Check sheet for the modelled part. Datum: model origin and axes. Units: mm. A direction names the side the tool comes from. Give positions to 0.01 mm unless a question says otherwise; leave off trailing zeros. Order: outer loops, then holes, each group sorted by start corner. A loop starts at its lowest first (then second) coordinate and runs counter-clockwise, first axis right, second up. Notation, with made-up numbers: M 28,-5.75 L 37,-5.75 A13 cw 37,14.25 Z; hole C 26,76.25 d2. An arc over 180 degrees is marked long. Answer in a Markdown table with one row per item. Add a question column.
from build123d import *

# Parameters (mm, degrees)
SKETCH2_W           = 57.5
SKETCH2_H           = 38
SKETCH2_W_2         = 47.5
SKETCH2_H_2         = 28
BOSS_EXTRUDE1_DEPTH = 2
SKETCH3_W           = 57.5
SKETCH3_H           = 38
SKETCH3_W_2         = 53.5
SKETCH3_H_2         = 34
BOSS_EXTRUDE2_DEPTH = 50
FILLET1_R           = 3
FILLET2_R           = 5
SKETCH4_W           = 15
SKETCH4_H           = 4
CUT_EXTRUDE1_DEPTH  = 2
FILLET3_R           = 3
CHAMFER1_SIZE       = 1
SKETCH6_W           = 15
SKETCH6_H           = 8
SKETCH6_R           = 1.75
BOSS_EXTRUDE3_DEPTH = 2.5
FILLET4_R           = 3


with BuildPart() as part:
    # Sketch2 → Boss-Extrude1 (new body)
    with BuildSketch(Plane(origin=(0, 0, 0), x_dir=(1, 0, 0), z_dir=(0, 1, 0))):
        Rectangle(SKETCH2_W, SKETCH2_H)
        Rectangle(SKETCH2_W_2, SKETCH2_H_2, mode=Mode.SUBTRACT)
    extrude(amount=BOSS_EXTRUDE1_DEPTH)

    # Sketch3 → Boss-Extrude2 (add)
    with BuildSketch(Plane.XZ):
        Rectangle(SKETCH3_W, SKETCH3_H)
        Rectangle(SKETCH3_W_2, SKETCH3_H_2, mode=Mode.SUBTRACT)
    extrude(amount=BOSS_EXTRUDE2_DEPTH)

    # Fillet1
    fillet1_edges = [part.edges().sort_by_distance(p)[0] for p in [
        (26.75, -25, -17),
        (26.75, -25, 17),
        (-26.75, -25, 17),
        (-26.75, -25, -17),
    ]]
    fillet(fillet1_edges, radius=FILLET1_R)

    # Fillet2
    fillet2_edges = [part.edges().sort_by_distance(p)[0] for p in [
        (28.75, -24, 19),
        (-28.75, -24, 19),
        (-28.75, -24, -19),
        (28.75, -24, -19),
    ]]
    fillet(fillet2_edges, radius=FILLET2_R)

    # Sketch4 → Cut-Extrude1 (cut)
    with BuildSketch(Plane.XY.offset(19)):
        with Locations((0, -48)):
            Rectangle(SKETCH4_W, SKETCH4_H)
    extrude(amount=-CUT_EXTRUDE1_DEPTH, mode=Mode.SUBTRACT)

    # Fillet3
    fillet3_edges = [part.edges().sort_by_distance(p)[0] for p in [
        (7.5, -46, 18),
        (-7.5, -46, 18),
    ]]
    fillet(fillet3_edges, radius=FILLET3_R)

    # Chamfer1
    chamfer1_edges = [part.edges().sort_by_distance(p)[0] for p in [
        (0, 2, 19),
        (-28.75, 2, 0),
        (28.75, 2, 0),
        (0, 2, -19),
        (27.285533906, 2, 17.535533906),
        (27.285533906, 2, -17.535533906),
        (-27.285533906, 2, -17.535533906),
        (-27.285533906, 2, 17.535533906),
    ]]
    chamfer(chamfer1_edges, length=CHAMFER1_SIZE)

    # Sketch6 → Boss-Extrude3 (add)
    with BuildSketch(Plane.XZ.offset(50)):
        with Locations((-21.25, 0)):
            Rectangle(SKETCH6_W, SKETCH6_H)
        with Locations((-18.75, 0)):
            Circle(SKETCH6_R, mode=Mode.SUBTRACT)
    boss_extrude3 = extrude(amount=-BOSS_EXTRUDE3_DEPTH)

    # Mirror1: Boss-Extrude3 across plane
    add(boss_extrude3.mirror(Plane(origin=(0, 0, 0), x_dir=(0, 0, 1), z_dir=(1, 0, 0))))

    # Fillet4
    fillet4_edges = [part.edges().sort_by_distance(p)[0] for p in [
        (-26.75, -48.75, -4),
        (-26.75, -48.75, 4),
        (-13.75, -48.75, 4),
        (-13.75, -48.75, -4),
        (26.75, -48.75, 4),
        (26.75, -48.75, -4),
        (13.75, -48.75, -4),
        (13.75, -48.75, 4),
    ]]
    fillet(fillet4_edges, radius=FILLET4_R)


solid = part.part
Q1. Tool access check on faces 5 (the flat face through (-22, -47.5, 0)), 6 (the flat face through (-20, -49, -4)), 7 (the flat face through (0, -25, 17)). Record the directions out of +Z, -Z, +X, -X, +Y, -Y that give a thin tool (end or side, any length) a straight path to the whole face; none if there is none.
Q2. Cross-section at B-B (z = 0). Record the boundary of the cut face in (x, y), and give its area (4 significant figures).
Q3. Draft check along Z on faces 1 (the cylindrical face through (27.25, -24.86, -17.57)), 2 (the flat face through (28.75, -25, 0)), 3 (the flat face through (-13.75, -49, 0)), 4 (the cylindrical face through (27.25, -24.14, 17.57)). Enter one of: pulls with the +Z half, pulls with the -Z half, needs draft (parallel to the pull), parting line crosses it, or undercut.
Q4. Thickness scan on probe 1 along Z at (x, y) = (18.75, -48.25); probe 2 along X at (y, z) = (-31.5, -5); probe 3 along Z at (x, y) = (23.5, -41). Record the ranges inside material, lowest first.
Q5. Cross-section at C-C (x = 18.75). Record the boundary of the cut face in (y, z).
Q6. Go/stop test with flat-tipped pins: pin 1 (4 mm diameter, centred on x = 18, z = 1, fed in from +Y); pin 2 (0.8 mm diameter, centred on y = -49.5, z = 18, fed in from +X); pin 3 (14.5 mm diameter, centred on x = 19.5, z = 2.5, fed in from +Y); pin 4 (0.5 mm diameter, centred on y = -49.5, z = 18, fed in from -X). Record where each tip stops, or that it passes through.
Q7. Cross-section at A-A (z = -8). Record the boundary of the cut face in (x, y), and give its area (3 significant figures).
Q8. Cross-section at D-D (y = -26). Record the boundary of the cut face in (x, z), and give its area (3 significant figures).
Values follow:
| question | item | result |
|---|---|---|
| 1 | face 5 | none |
| 1 | face 6 | +Y, -Y |
| 1 | face 7 | -Y |
| 2 | outline | M -28.75,-50 L -20.5,-50 L -20.5,-47.5 L -26.75,-47.5 L -26.75,0 L -23.75,0 L -23.75,2 L -27.75,2 L -28.75,1 Z; M -17,-50 L -13.75,-50 L -13.75,-47.5 L -17,-47.5 Z; M 13.75,-50 L 17,-50 L 17,-47.5 L 13.75,-47.5 Z; M 20.5,-50 L 28.75,-50 L 28.75,1 L 27.75,2 L 23.75,2 L 23.75,0 L 26.75,0 L 26.75,-47.5 L 20.5,-47.5 Z |
| 2 | area | 266.5 mm² |
| 3 | face 1 | pulls with the -Z half |
| 3 | face 2 | needs draft |
| 3 | face 3 | undercut |
| 3 | face 4 | pulls with the +Z half |
| 4 | probe 1 | -19 to -17, -4 to -1.75, 1.75 to 4, 17 to 19 |
| 4 | probe 2 | -28.75 to -26.75, 26.75 to 28.75 |
| 4 | probe 3 | -19 to -17, 17 to 19 |
| 5 | outline | M -50,-19 L 1,-19 L 2,-18 L 2,-14 L 0,-14 L 0,-17 L -50,-17 Z; M -50,-4 L -47.5,-4 L -47.5,-1.75 L -50,-1.75 Z; M -50,1.75 L -47.5,1.75 L -47.5,4 L -50,4 Z; M -50,17 L 0,17 L 0,14 L 2,14 L 2,18 L 1,19 L -50,19 Z |
| 6 | pin 1 | y = -47.5 |
| 6 | pin 2 | x = 27.22 |
| 6 | pin 3 | y = 2 |
| 6 | pin 4 | x = -27.06 |
| 7 | outline | M -28.75,-50 L -26.75,-50 L -26.75,0 L -23.75,0 L -23.75,2 L -27.75,2 L -28.75,1 Z; M 23.75,0 L 26.75,0 L 26.75,-50 L 28.75,-50 L 28.75,1 L 27.75,2 L 23.75,2 Z |
| 7 | area | 219 mm² |
| 8 | outline | M -28.75,-14 A5 ccw -23.75,-19 L 23.75,-19 A5 ccw 28.75,-14 L 28.75,14 A5 ccw 23.75,19 L -23.75,19 A5 ccw -28.75,14 Z; hole M -26.75,-14 A3 ccw -23.75,-17 L 23.75,-17 A3 ccw 26.75,-14 L 26.75,14 A3 ccw 23.75,17 L -23.75,17 A3 ccw -26.75,14 Z |
| 8 | area | 352 mm² |
